For this review, use the dimensioned drawing (mm, ordinates from the lowest corner) and the shaded views. A direction names the side the tool comes from. Coordinates: 2 decimals unless noted, no trailing zeros. Loops run counter-clockwise (first coordinate to the right, second up) from the corner with the lowest first, then second, coordinate; pieces in that order, holes last. Notation, with made-up numbers: (25, 84.25) - (57, 84.25) arc R17 cw to (57, 109.25) - close; hole circle Ø1 at (74, 59). An arc over 180 degrees is marked (long way). One line per item, written item: value. Start each with the question number.
1. To check wall thickness, follow line 1 (Y direction, x = 19.05, z = 7.5); line 2 (Z direction, x = 4.5, y = 5.75) (1 decimal); line 3 (Y direction, x = 2.15, z = 40). State the ranges of each line that lie inside material, in increasing order.
2. We need section A-A, the plane y = 4.5. Give the boundary of the cut face in (x, z), then the cut area to 3 significant figures.
3. Insertion check: P1, Ø2.5, axis at y = 7.5, z = 40, coming from the +X side; P2, Ø4, axis at y = 5.5, z = 26, coming from the +X side; P3, Ø2, axis at y = 7.5, z = 7.5, coming from the +X side; P4, Ø1, axis at x = 10.5, y = 13.5, coming from the +Z side. Each pin has a flat end and moves straight along its axis. Give the tip position at first contact, or say it passes through.
4. We need section D-D, the plane z = 7.5. Give the boundary of the cut face in (x, y).
5. Mouldability with a two-part tool opening along Z and no side actions: class the marked faces 3, 4, 5 and 6 as +Z half, -Z half, draft (parallel to the pull), parting line (faces both ways), or undercut.
6. For the marked faces 1 and 2, list the 3-axis set-ups (+Z, -Z, +X, -X, +Y, -Y) from which the entire face can be reached by the end or side of a thin tool; tool diameter is ignored.
7. We need section C-C, the plane x = 8.25. Give the boundary of the cut face in (y, z), then the cut area to 3 significant figures.
8. We need section B-B, the plane z = 32.5. Give the boundary of the cut face in (x, y).
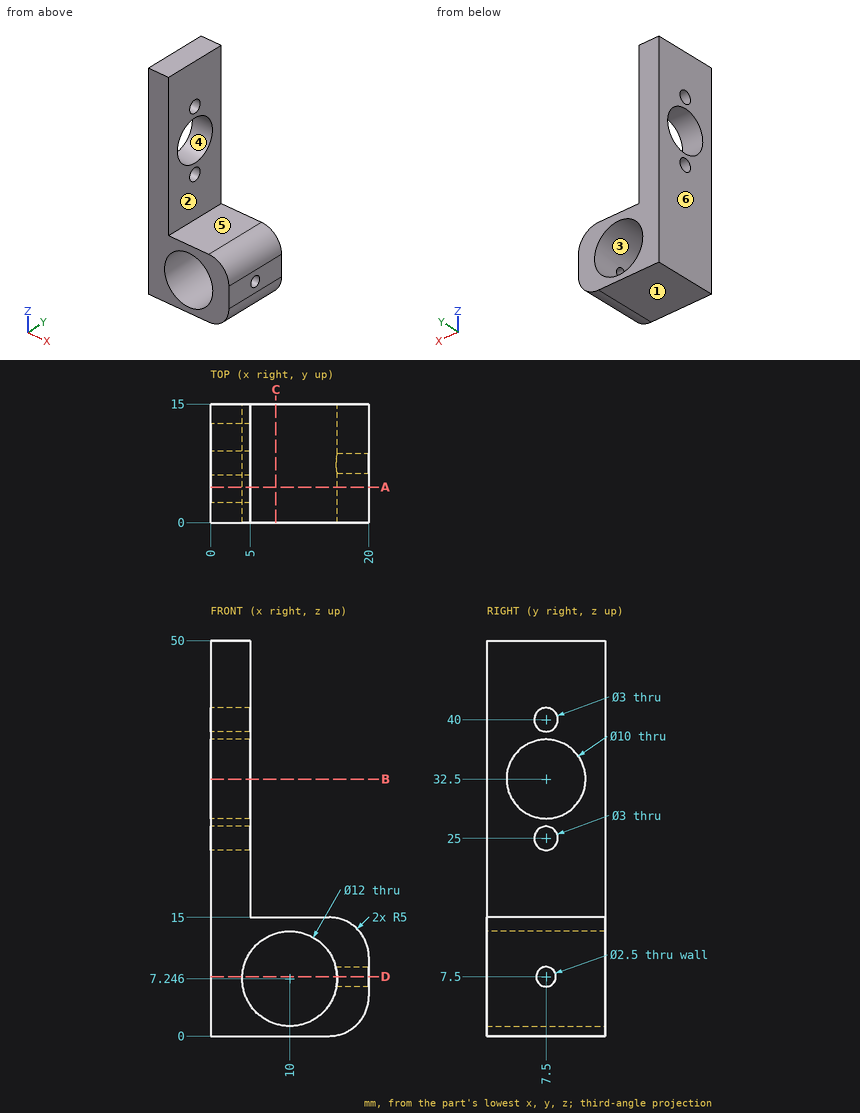
Findings below:
1. line 1: 0 to 6.25, 8.75 to 15
1. line 2: 0 to 4.8, 9.6 to 27.8, 37.2 to 50
1. line 3: 0 to 6, 9 to 15
2. outline: (0, 0) - (15, 0) arc R5 ccw to (20, 5) - (20, 10) arc R5 ccw to (15, 15) - (5, 15) - (5, 28.5) - (0, 28.5) - close; (0, 36.5) - (5, 36.5) - (5, 50) - (0, 50) - close; hole circle Ø12 at (10, 7.25)
2. area: 311 mm2
3. P1: through
3. P2: x = 5
3. P3: x = 4.13
3. P4: z = 15
4. outline: (0, 0) - (4.01, 0) - (4.01, 15) - (0, 15) - close; (15.99, 0) - (20, 0) - (20, 6.25) - (15.99, 6.25) - close; (15.99, 8.75) - (20, 8.75) - (20, 15) - (15.99, 15) - close
5. face 3: undercut
5. face 4: undercut
5. face 5: +Z half
5. face 6: draft
6. face 1: -Z, +X, -X, +Y, -Y
6. face 2: +Z, +X, +Y, -Y
7. outline: (0, 0) - (15, 0) - (15, 1.51) - (0, 1.51) - close; (0, 12.99) - (15, 12.99) - (15, 15) - (0, 15) - close
7. area: 52.8 mm2
8. outline: (0, 0) - (5, 0) - (5, 2.5) - (0, 2.5) - close; (0, 12.5) - (5, 12.5) - (5, 15) - (0, 15) - close
